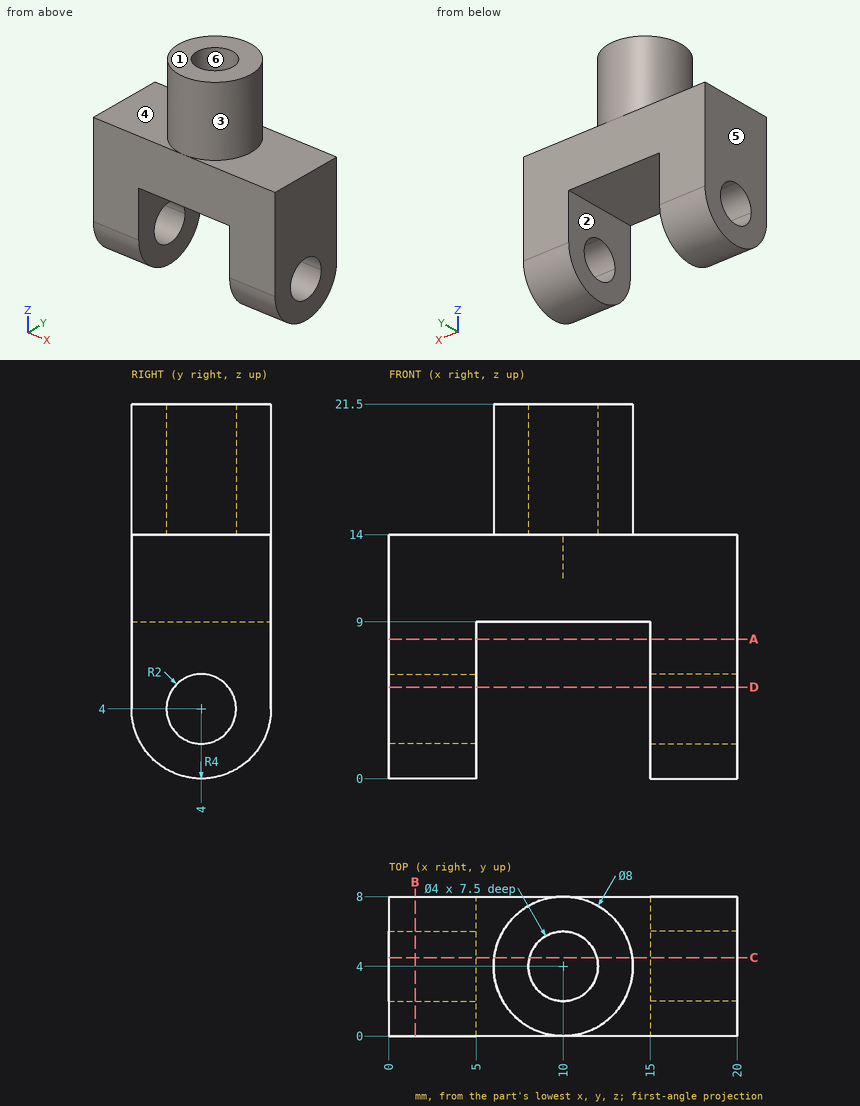
The figure shows three views and two pictorial views of one solid part (mm, origin at its lowest corner). Answer the questions. A direction names the side the tool comes from. Give positions to 0.01 mm unless a question says otherwise; leave off trailing zeros. Order: outer loops, then holes, each group sorted by start corner. A loop starts at its lowest first (then second) coordinate and runs counter-clockwise, first axis right, second up. Notation, with made-up numbers: (-27, 44) -> (24, 44) arc R3 cw to (24, 48) -> close; hole circle Ø3 at (-30, -40). An arc over 180 degrees is marked (long way). Answer as a JSON object with one key per item and string values. Group by question number.
Item 1: The part is cut by section D-D on z = 5.25. Write down the section's boundary in (x, y).
Item 2: Flat-ended cylindrical pins translate along their axes: pin 1 (2.5 mm diameter, centred on x = 2.5, y = 6, fed in from +Z); pin 2 (3 mm diameter, centred on x = 10, y = 4, fed in from -Z); pin 3 (4 mm diameter, centred on y = 3.5, z = 19, fed in from -X). Find the tip coordinate at first contact, or state that the pin passes through.
Item 3: Consider L1, parallel to X at y = 4, z = 18; L2, parallel to X at y = 6, z = 8; L3, parallel to Y at x = 10, z = 15.5. Determine where each line is inside the solid, lowest interval first. Write a range as from..to.
Item 4: The part is cut by section A-A on z = 8. Write down the section's boundary in (x, y), and give its area (3 significant figures).
Item 5: The part is cut by section B-B on x = 1.5. Write down the section's boundary in (y, z), and give its area (3 significant figures).
Item 6: The part is cut by section C-C on y = 4.5. Write down the section's boundary in (x, z), and give its area (3 significant figures).
Item 7: Determine the mould class of the marked faces 4, 5 and 6 for opening direction X: pulls with the +X half, pulls with the -X half, needs draft (parallel to the pull), parting line crosses it, or undercut.
Item 8: A tool of negligible diameter and unlimited length cuts with its end or side. For the marked faces 1, 2 and 3, from which of +Z, -Z, +X, -X, +Y, -Y can it reach the whole face along a straight path? Write none if from no direction.
Result set:
{
 "1": {"outline": "(0, 0) -> (5, 0) -> (5, 2.44) -> (0, 2.44) -> close; (0, 5.56) -> (5, 5.56) -> (5, 8) -> (0, 8) -> close; (15, 0) -> (20, 0) -> (20, 2.44) -> (15, 2.44) -> close; (15, 5.56) -> (20, 5.56) -> (20, 8) -> (15, 8) -> close"},
 "2": {"pin 1": "z = 14", "pin 2": "z = 9", "pin 3": "x = 6"},
 "3": {"L1": "6..8, 12..14", "L2": "0..5, 15..20", "L3": "0..2, 6..8"},
 "4": {"outline": "(0, 0) -> (5, 0) -> (5, 8) -> (0, 8) -> close; (15, 0) -> (20, 0) -> (20, 8) -> (15, 8) -> close", "area": "80.0 mm²"},
 "5": {"outline": "(0, 4) arc R4 ccw to (8, 4) -> (8, 14) -> (0, 14) -> close; hole circle Ø4 at (4, 4)", "area": "92.6 mm²"},
 "6": {"outline": "(0, 0.03) -> (5, 0.03) -> (5, 2.06) -> (0, 2.06) -> close; (0, 5.94) -> (5, 5.94) -> (5, 9) -> (15, 9) -> (15, 5.94) -> (20, 5.94) -> (20, 14) -> (13.97, 14) -> (13.97, 21.5) -> (11.94, 21.5) -> (11.94, 14) -> (8.06, 14) -> (8.06, 21.5) -> (6.03, 21.5) -> (6.03, 14) -> (0, 14) -> close; (15, 0.03) -> (20, 0.03) -> (20, 2.06) -> (15, 2.06) -> close", "area": "181 mm²"},
 "7": {"face 4": "needs draft", "face 5": "pulls with the -X half", "face 6": "undercut"},
 "8": {"face 1": "+Z, +X, -X, +Y, -Y", "face 2": "-Z, +Y, -Y", "face 3": "+Z"}
}
